```python
from build123d import *

# Parameters (mm, degrees)
SKETCH3_R         = 5.861538462
GEARBODY_DEPTH    = 6.096
TOOTHCUT_DEPTH    = 11.289629841
CIRPATTERN1_COUNT = 10
BOREDIA_R         = 1.27
BORE_DEPTH        = 12700


with BuildPart() as part:
    # Sketch3 → gearBody (new body)
    with BuildSketch(Plane.XY):
        with Locations(Location((0, 0, 0), (0, 0, 180))):
            Circle(SKETCH3_R)
    extrude(amount=GEARBODY_DEPTH)

    # Sketch2 → toothCut (cut, through all)
    with BuildSketch(Plane.XY):
        with BuildLine():
            ThreePointArc((3.410371072, -1.3326694), (3.459525577, -1.199300364), (3.503466664, -1.064124012))
            ThreePointArc((3.503466664, -1.064124012), (3.673182044, -0.842791414), (3.946639633, -0.787906299))
            ThreePointArc((3.946639633, -0.787906299), (5.609569592, -0.511317374), (6.763505117, 0.717613171))
            ThreePointArc((6.763505117, 0.717613171), (6.426274445, -2.22777173), (4.868104082, -4.749898186))
            ThreePointArc((4.868104082, -4.749898186), (4.722411681, -3.07043065), (3.587488494, -1.823920787))
            ThreePointArc((3.587488494, -1.823920787), (3.406677364, -1.61155609), (3.410371072, -1.3326694))
        make_face()
    toothcut = extrude(amount=TOOTHCUT_DEPTH, mode=Mode.SUBTRACT)

    # CirPattern1: toothCut ×10 about axis
    cirpattern1_axis = Axis((0, 0, 0), (0, 0, 1))
    for i in range(1, CIRPATTERN1_COUNT):
        add(toothcut.rotate(cirpattern1_axis, i * 360 / CIRPATTERN1_COUNT), mode=Mode.SUBTRACT)

    # boreDia → bore (cut, symmetric)
    with BuildSketch(Plane.XY):
        Circle(BOREDIA_R)
    extrude(amount=BORE_DEPTH, both=True, mode=Mode.SUBTRACT)


solid = part.part
```
Work out the finished part from the listing and answer in its coordinate system (mm). A direction names the side the tool comes from. Give positions to 0.01 mm unless a question says otherwise; leave off trailing zeros. Loops run counter-clockwise (first coordinate to the right, second up) from the corner with the lowest first, then second, coordinate; pieces in that order, holes last. Notation, with made-up numbers: (77.25, -5.75) - (101.25, -5.75) arc R8 ccw to (101.25, 1.25) - close; hole circle Ø3 at (28, 75). An arc over 180 degrees is marked (long way). Use CSV: the item, a comma, the result in double quotes. Start each with the question number.
(1) A tool of negligible diameter and unlimited length cuts with its end or side. For faces 1 (the face through (3.697, 3.381, 3.005)), 2 (the face through (4.433, 2.278, 3.005)), 3 (the face through (-1, -4.9, 3)), 4 (the face through (4.93, -0.76, 3.01)), from which of +Z, -Z, +X, -X, +Y, -Y can it reach the whole face along a straight path? Write none if from no direction.
(2) Find section B-B, the plane y = 5. Determine the outline of the cut face in (x, z).
(3) Find section A-A, the plane x = -4.25. Determine the outline of the cut face in (y, z), plus the area to 3 significant figures.
(4) Find section C-C, the plane x = 5.25. Determine the outline of the cut face in (y, z).
(5) Determine the mould class of faces 5 (the face through (3.536, -3.512, 3.005)), 6 (the face through (2.073, -4.561, 3.005)), 7 (the face through (1, 4.9, 3)) for opening direction Y: released by +Y, released by -Y, zero draft, split by the parting line, or undercut.
(6) This flat-tipped pin is pushed along its axis until it touches: pin 1 (1 mm diameter, centred on x = 0.5, z = 3, fed in from -Y). Where does it stop, or does it pass through?
(7) Find the intervals of material crossed by L1, parallel to Y at x = 0, z = 2; L2, parallel to Y at x = -4.25, z = 0.75; L3, parallel to Y at x = -4, z = 5, in increasing order.
(8) Find section D-D, the plane y = 2. Determine the outline of the cut face in (x, z), plus the area to 3 significant figures.
Results found:
1,face 1,"+Z, -Z, +Y"
1,face 2,"+Z, -Z, +X"
1,face 3,"+Z, -Z, -Y"
1,face 4,"+Z, -Z"
2,outline,"(-2.06, 0) - (-0.85, 0) - (-0.85, 6.1) - (-2.06, 6.1) - close; (1.07, 0) - (2.25, 0) - (2.25, 6.1) - (1.07, 6.1) - close"
3,outline,"(-3.53, 0) - (-2.09, 0) - (-2.09, 6.1) - (-3.53, 6.1) - close; (-0.65, 0) - (0.82, 0) - (0.82, 6.1) - (-0.65, 6.1) - close; (2.35, 0) - (3.71, 0) - (3.71, 6.1) - (2.35, 6.1) - close"
3,area,"26.0 mm^2"
4,outline,"(-0.67, 0) - (0.47, 0) - (0.47, 6.1) - (-0.67, 6.1) - close"
5,face 5,"released by -Y"
5,face 6,"undercut"
5,face 7,"released by +Y"
6,pin 1,"y = -5.22"
7,L1,"-3.66 to -1.27, 1.27 to 3.66"
7,L2,"-3.53 to -2.09, -0.65 to 0.82, 2.35 to 3.71"
7,L3,"-3.48 to -1.89, -0.64 to 0.8, 2.11 to 3.67"
8,outline,"(-3.86, 0) - (4.14, 0) - (4.14, 6.1) - (-3.86, 6.1) - close"
8,area,"48.8 mm^2"
